Here's the drawing with two shaded views (mm, measured from the low corner). I have some questions. Round coordinates to 2 decimals unless told otherwise and drop trailing zeros. Order: outer loops, then holes, each group sorted by start corner. A loop starts at its lowest first (then second) coordinate and runs counter-clockwise, first axis right, second up.
Q1. If we section it at A-A (z = 50.5): Please give me the cut outline in (x, y), plus the area to 3 significant figures.
Q2. Will these pins go through, and if not, where does the flat tip stop? P1, Ø0.9, axis at x = 242, y = 1, coming from the +Z side; P2, Ø0.9, axis at y = 1, z = 82.5, coming from the +X side; P3, Ø0.9, axis at x = 2, y = 1.5, coming from the -Z side.
Q3. If we section it at B-B (z = 9): Please give me the cut outline in (x, y).
Q4. If I drill on line 1 (X direction, y = 2.25, z = 43.5); line 2 (X direction, y = 0.8, z = 32); line 3 (X direction, y = 1.25, z = 55.5), over which ranges is the centre line in solid material (lowest first)?
Q5. If we section it at D-D (z = 33.5): Please give me the cut outline in (x, y), plus the area to 3 significant figures.
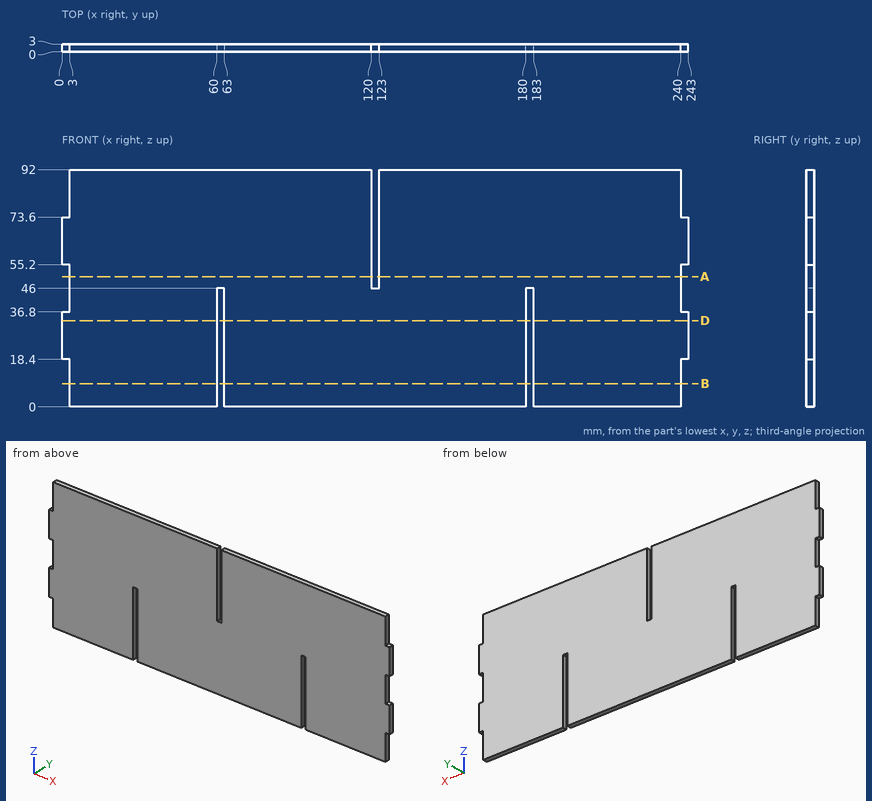
Solution:
1. outline: (3, 0) - (120, 0) - (120, 3) - (3, 3) - close; (123, 0) - (240, 0) - (240, 3) - (123, 3) - close
1. area: 702 mm2
2. P1: stops at z = 73.6
2. P2: stops at x = 240
2. P3: stops at z = 18.4
3. outline: (3, 0) - (60, 0) - (60, 3) - (3, 3) - close; (63, 0) - (180, 0) - (180, 3) - (63, 3) - close; (183, 0) - (240, 0) - (240, 3) - (183, 3) - close
4. line 1: x = 3 to 60, 63 to 180, 183 to 240
4. line 2: x = 0 to 60, 63 to 180, 183 to 243
4. line 3: x = 0 to 120, 123 to 243
5. outline: (0, 0) - (60, 0) - (60, 3) - (0, 3) - close; (63, 0) - (180, 0) - (180, 3) - (63, 3) - close; (183, 0) - (243, 0) - (243, 3) - (183, 3) - close
5. area: 711 mm2
